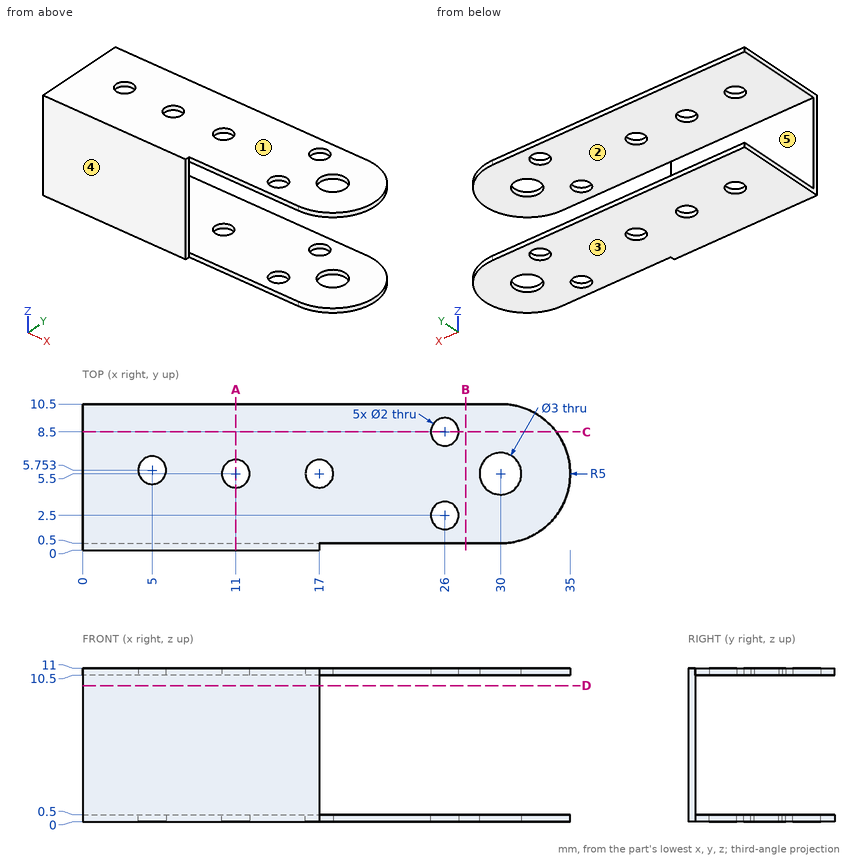
Input: dimensioned drawing with shaded views. Units: mm. Origin: part minimum x, y, z. A direction names the side the tool comes from. Coordinates: 2 decimals unless noted, no trailing zeros. Loops run counter-clockwise (first coordinate to the right, second up) from the corner with the lowest first, then second, coordinate; pieces in that order, holes last. Notation, with made-up numbers: (-34.5, -5.5) -> (-12.5, -5.5) arc R26 ccw to (-12.5, 25.5) -> close; hole circle Ø8 at (-39.75, -8). An arc over 180 degrees is marked (long way). One line per item, written item: value. Start each with the question number.
Q1. Section query A-A, the plane x = 11. Return the cut outline in (y, z).
Q2. Mould query, pull axis Z, two halves, no side actions, for the marked faces 1, 2 and 3. Classes: pulls with the +Z half, pulls with the -Z half, needs draft (parallel to the pull), parting line crosses it, or undercut.
Q3. Section query C-C, the plane y = 8.5. Return the cut outline in (x, z).
Q4. Line query: line 1 along Z through (x, y) = (5, 1.25); line 2 along Y through (x, z) = (26, 0.3); line 3 along Y through (x, z) = (30, 0.45). Output: solid intervals per line, ascending.
Q5. Section query D-D, the plane z = 9.75. Return the cut outline in (x, y).
Q6. Set-up query: the marked faces 4 and 5. Return all of +Z, -Z, +X, -X, +Y, -Y with unobstructed straight access to the full face (end or side cutting, diameter ignored); none if empty.
Q7. Section query B-B, the plane x = 27.5. Return the cut outline in (y, z), and give its area (3 significant figures).
Q8. Contact query for flat-ended pins moving along their axis: P1, Ø1.2, axis at x = 11, y = 5.5, coming from the +Z side; P2, Ø5, axis at x = 6, z = 5.5, coming from the +Y side. Output: stop coordinate, or through.
Results:
1. outline: (0, 0) -> (4.5, 0) -> (4.5, 0.5) -> (0.5, 0.5) -> (0.5, 10.5) -> (4.5, 10.5) -> (4.5, 11) -> (0, 11) -> close; (6.5, 0) -> (10.5, 0) -> (10.5, 0.5) -> (6.5, 0.5) -> close; (6.5, 10.5) -> (10.5, 10.5) -> (10.5, 11) -> (6.5, 11) -> close
2. face 1: pulls with the +Z half
2. face 2: undercut
2. face 3: pulls with the -Z half
3. outline: (0, 0) -> (25, 0) -> (25, 0.5) -> (0, 0.5) -> close; (0, 10.5) -> (25, 10.5) -> (25, 11) -> (0, 11) -> close; (27, 0) -> (34, 0) -> (34, 0.5) -> (27, 0.5) -> close; (27, 10.5) -> (34, 10.5) -> (34, 11) -> (27, 11) -> close
4. line 1: 0 to 0.5, 10.5 to 11
4. line 2: 0.5 to 1.5, 3.5 to 7.5, 9.5 to 10.5
4. line 3: 0.5 to 4, 7 to 10.5
5. outline: (0, 0) -> (17, 0) -> (17, 0.5) -> (0, 0.5) -> close
6. face 4: +Z, -Z, +X, -X, -Y
6. face 5: +X, -X, +Y
7. outline: (0.5, 0) -> (10.5, 0) -> (10.5, 0.5) -> (0.5, 0.5) -> close; (0.5, 10.5) -> (10.5, 10.5) -> (10.5, 11) -> (0.5, 11) -> close
7. area: 10.0 mm^2
8. P1: through
8. P2: y = 0.5
